Drawing for the job (mm, zero at the part's lowest x, y, z). A direction names the side the tool comes from. Give positions to 0.01 mm unless a question says otherwise; leave off trailing zeros. Order: outer loops, then holes, each group sorted by start corner. A loop starts at its lowest first (then second) coordinate and runs counter-clockwise, first axis right, second up. Notation, with made-up numbers: (7.5, -2.75) - (61.5, -2.75) arc R26 ccw to (61.5, 24.25) - close; hole circle Ø4 at (17.5, 29). An arc over 180 degrees is marked (long way). One line per item, written item: value.
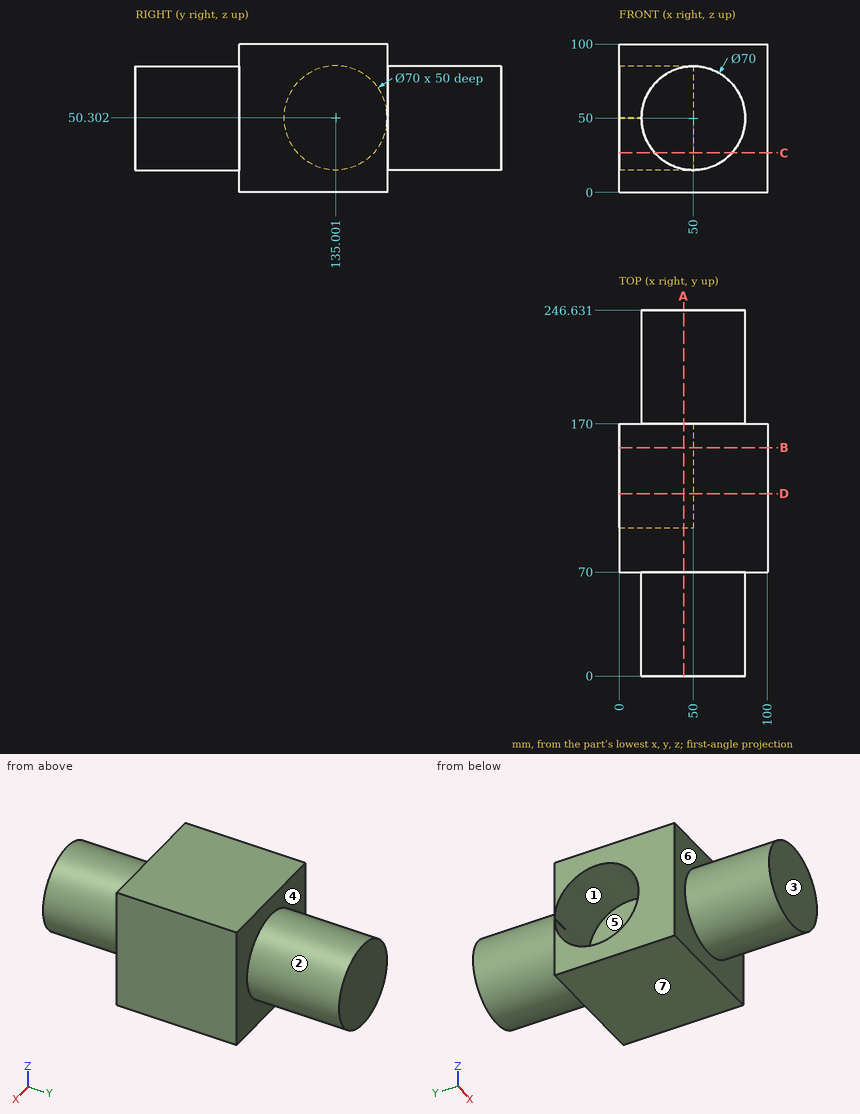
(1) Drill centre lines: line 1 (Y direction, x = 30, z = 51.5); line 2 (X direction, y = 197, z = 49.5); line 3 (Y direction, x = 58, z = 92.5). Where is each one in solid material? Low to high.
Completed:
line 1: 0 to 100.02, 169.98 to 246.63
line 2: 15 to 85
line 3: 70 to 170
(2) Slice it at B-B, the plane y = 154. Give the cut face in (x, z).
Completed:
outline: (0, 0) - (100, 0) - (100, 100) - (0, 100) - (0, 79.7) - (50, 79.7) - (50, 20.91) - (0, 20.91) - close
(3) Slice it at A-A, the plane x = 43.5. Give the cut face in (y, z).
Completed:
outline: (0, 15.61) - (70, 15.61) - (70, 0) - (170, 0) - (170, 15.61) - (246.63, 15.61) - (246.63, 84.39) - (170, 84.39) - (170, 100) - (70, 100) - (70, 84.39) - (0, 84.39) - close; hole circle Ø70 at (135, 50.3)
(4) Pin check, flat tips, straight feed: P1, Ø12, axis at x = 54, z = 87.5, coming from the +Y side; P2, Ø1, axis at x = 65.5, y = 187.5, coming from the -Z side; P3, Ø4, axis at y = 141.5, z = 64.5, coming from the -X side; P4, Ø8, axis at x = 19.5, z = 23.5, coming from the +Y side. Stop position of each tip, or through.
Completed:
P1: y = 246.63
P2: z = 18.38
P3: x = 50
P4: y = 170
(5) 3-axis set-ups, long thin cutter, end or side, ignore diameter. For the marked faces 5, 6 and 7: which of +Z, -Z, +X, -X, +Y, -Y reach the whole face in a straight line?
Completed:
face 5: -X
face 6: -Y
face 7: -Z, +X, -X, +Y, -Y
(6) Slice it at D-D, the plane y = 123. Give the cut face in (x, z).
Completed:
outline: (0, 0) - (100, 0) - (100, 100) - (0, 100) - (0, 83.18) - (50, 83.18) - (50, 17.42) - (0, 17.42) - close
(7) Slice it at C-C, the plane z = 26.5. Give the cut face in (x, y).
Completed:
outline: (0, 70) - (24.06, 70) - (24.06, 0) - (75.94, 0) - (75.94, 70) - (100, 70) - (100, 170) - (75.94, 170) - (75.94, 246.63) - (24.06, 246.63) - (24.06, 170) - (0, 170) - (0, 160.66) - (50, 160.66) - (50, 109.34) - (0, 109.34) - close
(8) Pull direction Y, two halves, no side cores. Call the marked faces 1, 2, 3 and 4: +Y half, -Y half, draft (parallel to the pull), parting line (faces both ways), or undercut.
Completed:
face 1: undercut
face 2: draft
face 3: -Y half
face 4: +Y half
